Geometry check sheet. Reference: drawing and pictorial views, mm from the part's lowest x, y, z. A direction names the side the tool comes from. Coordinates: 2 decimals unless noted, no trailing zeros. Write each loop counter-clockwise with the first axis right and the second up, starting at its lowest first coordinate (ties: lowest second). Pieces come first, ordered by that corner, then holes. Notation, with made-up numbers: (10.25, 42) -> (52.25, 42) arc R22 cw to (52.25, 72) -> close; hole circle Ø2 at (56.5, 7). An arc over 180 degrees is marked (long way). Use a Markdown table: item, result.
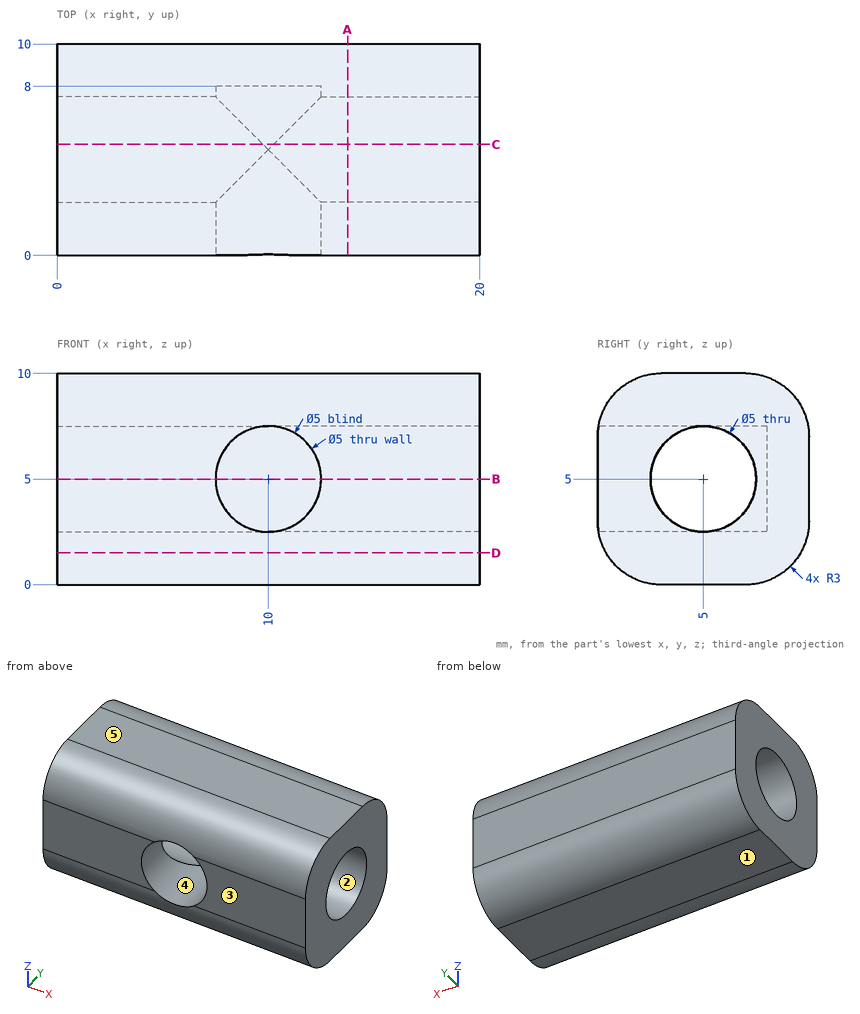
Item 1: Depth check by flat-ended pin: P1, Ø3, axis at x = 8, z = 2.5, coming from the +Y side. Enter the tip coordinate at first touch or a pass-through.
Answer block:
| item | result |
|---|---|
| P1 | stops at y = 10 |
Item 2: Mould release check, pull along Z, two halves, no side actions. Record for the marked faces 1, 2 and 3: +Z half, -Z half, draft (parallel to the pull), parting line (faces both ways), or undercut.
Answer block:
| item | result |
|---|---|
| face 1 | -Z half |
| face 2 | undercut |
| face 3 | draft |
Item 3: Section check D-D on z = 1.5. Record the boundary of the cut face in (x, y), then the cut area to 3 significant figures.
Answer block:
| item | result |
|---|---|
| outline | (0, 0.4) -> (20, 0.4) -> (20, 9.6) -> (0, 9.6) -> close |
| area | 184 mm^2 |
Item 4: Thickness scan on L1, parallel to Z at x = 13.75, y = 5; L2, parallel to Z at x = 4, y = 3.5; L3, parallel to X at y = 1, z = 3. Record the ranges inside material, lowest first. Write a range as [from, to].
Answer block:
| item | result |
|---|---|
| L1 | z = [0, 2.5], [7.5, 10] |
| L2 | z = [0, 3], [7, 10] |
| L3 | x = [0, 8.5], [11.5, 20] |
Item 5: Tool access check on the marked faces 4 and 5. Record the directions out of +Z, -Z, +X, -X, +Y, -Y that give a thin tool (end or side, any length) a straight path to the whole face; none if there is none.
Answer block:
| item | result |
|---|---|
| face 4 | -Y |
| face 5 | +Z, +X, -X, +Y, -Y |
Item 6: Section check B-B on z = 5. Record the boundary of the cut face in (x, y), then the cut area to 3 significant figures.
Answer block:
| item | result |
|---|---|
| outline | (0, 0) -> (7.5, 0) -> (7.5, 2.5) -> (0, 2.5) -> close; (0, 7.5) -> (7.5, 7.5) -> (7.5, 8) -> (12.5, 8) -> (12.5, 7.5) -> (20, 7.5) -> (20, 10) -> (0, 10) -> close; (12.5, 0) -> (20, 0) -> (20, 2.5) -> (12.5, 2.5) -> close |
| area | 85.0 mm^2 |
Item 7: Section check A-A on x = 13.75. Record the boundary of the cut face in (y, z).
Answer block:
| item | result |
|---|---|
| outline | (0, 3) arc R3 ccw to (3, 0) -> (7, 0) arc R3 ccw to (10, 3) -> (10, 7) arc R3 ccw to (7, 10) -> (3, 10) arc R3 ccw to (0, 7) -> close; hole circle Ø5 at (5, 5) |
Item 8: Section check C-C on y = 5.25. Record the boundary of the cut face in (x, z).
Answer block:
| item | result |
|---|---|
| outline | (0, 0) -> (20, 0) -> (20, 2.51) -> (10.25, 2.51) arc R2.5 cw to (9.75, 2.51) -> (0, 2.51) -> close; (0, 7.49) -> (9.75, 7.49) arc R2.5 cw to (10.25, 7.49) -> (20, 7.49) -> (20, 10) -> (0, 10) -> close |
